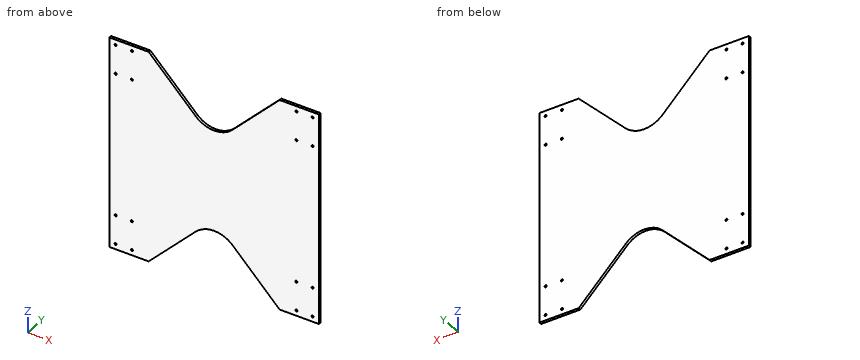
from build123d import *

# Parameters (mm, degrees)
SKETCH1_R           = 1.95
BOSS_EXTRUDE1_DEPTH = 5
FILLET1_R           = 50


with BuildPart() as part:
    # Sketch1 → Boss-Extrude1 (new body)
    with BuildSketch(Plane(origin=(0, 0, 0), x_dir=(1, 0, 0), z_dir=(0, 1, 0))):
        Polygon((-171.385103045, 78.719364296), (-46.385103045, 203.765478515), (28.614896955, 203.765478515), (28.614896955, 3.765478515), (28.707125389, -196.23450022), (-46.292866637, -196.269085883), (-171.350517383, -71.28062773), (-296.350517383, -196.326741949), (-371.350517383, -196.326741949), (-371.350517383, 3.673258051), (-371.442745817, 203.673236785), (-296.442753791, 203.707822448), align=None)
        with Locations((16.614896955, 193.765478515)):
            Circle(SKETCH1_R, mode=Mode.SUBTRACT)
        with Locations((-14.385103045, 193.765478515)):
            Circle(SKETCH1_R, mode=Mode.SUBTRACT)
        with Locations((-14.385103045, 138.925478515)):
            Circle(SKETCH1_R, mode=Mode.SUBTRACT)
        with Locations((16.614896955, 138.925478515)):
            Circle(SKETCH1_R, mode=Mode.SUBTRACT)
        with Locations((16.677226206, -131.40004082)):
            Circle(SKETCH1_R, mode=Mode.SUBTRACT)
        with Locations((-14.322770498, -131.414336227)):
            Circle(SKETCH1_R, mode=Mode.SUBTRACT)
        with Locations((16.702515243, -186.240034989)):
            Circle(SKETCH1_R, mode=Mode.SUBTRACT)
        with Locations((-14.297481461, -186.254330396)):
            Circle(SKETCH1_R, mode=Mode.SUBTRACT)
        with Locations((-328.350517383, -186.326741949)):
            Circle(SKETCH1_R, mode=Mode.SUBTRACT)
        with Locations((-359.350517383, -186.326741949)):
            Circle(SKETCH1_R, mode=Mode.SUBTRACT)
        with Locations((-328.350517383, -131.486741949)):
            Circle(SKETCH1_R, mode=Mode.SUBTRACT)
        with Locations((-359.350517383, -131.486741949)):
            Circle(SKETCH1_R, mode=Mode.SUBTRACT)
        with Locations((-359.412846634, 138.838777386)):
            Circle(SKETCH1_R, mode=Mode.SUBTRACT)
        with Locations((-328.41284993, 138.853072793)):
            Circle(SKETCH1_R, mode=Mode.SUBTRACT)
        with Locations((-328.438138967, 193.693066962)):
            Circle(SKETCH1_R, mode=Mode.SUBTRACT)
        with Locations((-359.438135671, 193.678771555)):
            Circle(SKETCH1_R, mode=Mode.SUBTRACT)
    extrude(amount=BOSS_EXTRUDE1_DEPTH)

    # Fillet1
    fillet1_edges = [part.edges().sort_by_distance(p)[0] for p in [
        (-171.385103045, 2.5, -78.719364296),
        (-171.350517383, 2.5, 71.28062773),
    ]]
    fillet(fillet1_edges, radius=FILLET1_R)


solid = part.part
Work out the finished part from the listing and answer in its coordinate system (mm). Give positions to 0.01 mm unless a question says otherwise; leave off trailing zeros. Loops run counter-clockwise (first coordinate to the right, second up) from the corner with the lowest first, then second, coordinate; pieces in that order, holes last. Notation, with made-up numbers: (-24.75, 45.5) -> (13.25, 45.5) arc R16 cw to (13.25, 59.5) -> close; hole circle Ø7 at (-34, 39.25). An arc over 180 degrees is marked (long way). Use a Markdown table: item, result. Add a question column.
1) The part is cut by section A-A, the plane z = 157.5. Determine the outline of the cut face in (x, y).
2) The part is cut by section B-B, the plane y = 1.6. Count the separate pieces of the cut face and the enclosed holes in it, plus the area to 3 significant figures.
3) The part is cut by section D-D, the plane z = -157. Determine the outline of the cut face in (x, y).
4) Each of these flat-tipped pins is pushed along its axis until it touches: P1, Ø2.5, axis at y = 1.5, z = 144.5, coming from the -X side; P2, Ø2, axis at x = -115.5, y = 1.5, coming from the +Z side; P3, Ø1.5, axis at y = 2.5, z = -129.5, coming from the +X side. Where does it stop, or does it pass through?
5) The part is cut by section C-C, the plane x = -280. Determine the outline of the cut face in (y, z).
6) Consider line 1 along X through (y, z) = (3, 49); line 2 along Z through (x, y) = (-305.5, 3.6); line 3 along Z through (x, y) = (-8.5, 2). Determine where each line is inside the solid, lowest interval first.
Reported:
| question | item | result |
|---|---|---|
| 1 | outline | (-371.35, 0) -> (-257.54, 0) -> (-257.54, 5) -> (-371.35, 5) -> close; (-85.08, 0) -> (28.69, 0) -> (28.69, 5) -> (-85.08, 5) -> close |
| 2 | separate pieces | 1 |
| 2 | enclosed holes | 16 |
| 2 | area | 130,000 mm^2 |
| 3 | outline | (-371.42, 0) -> (-249.71, 0) -> (-249.71, 5) -> (-371.42, 5) -> close; (-93.13, 0) -> (28.61, 0) -> (28.61, 5) -> (-93.13, 5) -> close |
| 4 | P1 | stops at x = -371.35 |
| 4 | P2 | stops at z = 128.1 |
| 4 | P3 | stops at x = 28.61 |
| 5 | outline | (0, -187.27) -> (5, -187.27) -> (5, 179.97) -> (0, 179.97) -> close |
| 6 | line 1 | x = -371.35 to 28.64 |
| 6 | line 2 | z = -203.7 to 196.33 |
| 6 | line 3 | z = -203.77 to 196.25 |
